Can you work these out from the model? Positions are in its coordinate system, mm. Face numbers are marked on the shaded views. Coordinates: 2 decimals unless noted, no trailing zeros. Write each loop counter-clockwise with the first axis right and the second up, starting at its lowest first coordinate (ties: lowest second). Pieces come first, ordered by that corner, then holes. Notation, with made-up numbers: (30, 29.5) -> (70, 29.5) arc R17 cw to (70, 56.5) -> close; hole circle Ø5 at (40, 20). An arc over 180 degrees is marked (long way). Use one line per item in the form item = value.
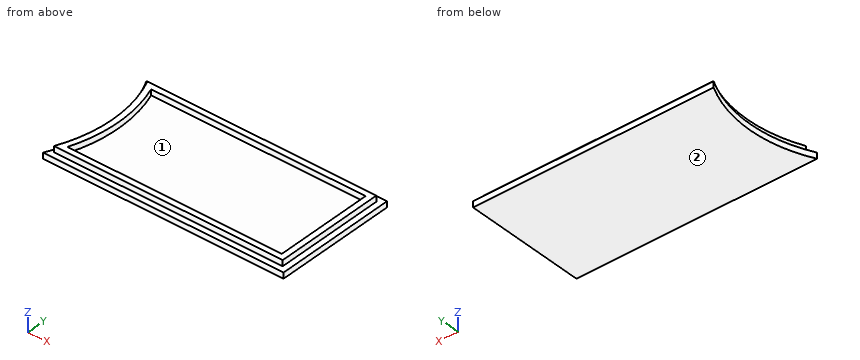
Autodesk Inventor part; units mm, degrees
ref_plane "YZ Plane" through (0, 0, 0) normal (1, 0, 0) x (0, 1, 0)
ref_plane "XZ Plane" through (0, 0, 0) normal (0, 1, 0) x (-1, 0, 0)
ref_plane "XY Plane" through (0, 0, 0) normal (0, 0, 1) x (1, 0, 0)
sketch "Sketch1" plane through (0, 0, 0) normal (0, 0, 1) x (1, 0, 0)
  circle A0 centre (0, 0) radius 45.75
  circle A1 centre (0, 0) radius 46.75
  line L0 (45.75, -0.0157) -> (46.75, -0.0157) construction
  line L1 (42.7149, 19) -> (121.75, 19)
  line L2 (121.75, 19) -> (121.75, -19)
  line L3 (121.75, -19) -> (42.7149, -19)
  line L4 (41.768, 21) -> (123.75, 21)
  line L5 (123.75, 21) -> (123.75, -21)
  line L6 (123.75, -21) -> (41.768, -21)
  line L7 (82.759, 21) -> (82.759, 19) construction
  line L8 (121.75, 0) -> (123.75, 0) construction
  line L9 (98.0367, -19) -> (98.0367, -21) construction
  line L10 (0, 0) -> (121.75, 0) construction
  line L11 (41.768, 21) -> (40.6456, 21)
  line L12 (41.768, -21) -> (40.6456, -21)
  line L13 (45.6899, 17) -> (119.75, 17)
  line L14 (119.75, 17) -> (119.75, -17)
  arc A2 (44.895, -19) -> (44.895, 19) centre (0, 0) ccw
  line L15 (119.75, -17) -> (45.6899, -17)
  dimension "d0" = 91.5
  dimension "d2" = 1
  dimension "d3" = 75
  dimension "d4" = 38
  dimension "d5" = 2
  dimension "d62" = 2
  dimension "d63" = 2
extrude "Extrusion13" add sketch "Sketch1" against normal blind 2 contours A0 L11 A1 L12 | L4 L5 L6 A1 L3 L2 L1 | L1 A2 L3 A1 | L1 L2 L3 A2 L15 L14 L13 | L13 L14 L15 A2 picked at (42.2726, -18.1004)
extrude "Extrusion14" add sketch "Sketch1" along normal blind 2 contours L1 A2 L3 A1 | L1 L2 L3 A2 L15 L14 L13
properties part number "Pump lid MM0312"
Q1. Will these pins go through, and if not, where does the flat tip stop? pin 1 (1 mm diameter, centred on x = 64.5, z = 1, fed in from -Y); pin 2 (12 mm diameter, centred on x = 105, y = 8, fed in from +Z); pin 3 (1.6 mm diameter, centred on y = -1, z = 1.5, fed in from -X).
Return value:
pin_1 = -19
pin_2 = 0
pin_3 = 46.72
Q2. Suppose I cut it at D-D (x = 48). Write out the boundary of the cut face in (y, z).
Return value:
outline = (-21, -2) -> (21, -2) -> (21, 0) -> (19, 0) -> (19, 2) -> (17, 2) -> (17, 0) -> (8.52, 0) -> (8.52, 2) -> (-8.52, 2) -> (-8.52, 0) -> (-17, 0) -> (-17, 2) -> (-19, 2) -> (-19, 0) -> (-21, 0) -> close
Q3. Suppose I cut it at A-A (x = 110). Write out the boundary of the cut face in (y, z).
Return value:
outline = (-21, -2) -> (21, -2) -> (21, 0) -> (19, 0) -> (19, 2) -> (17, 2) -> (17, 0) -> (-17, 0) -> (-17, 2) -> (-19, 2) -> (-19, 0) -> (-21, 0) -> close
Q4. Thinking about a two-plate mould opening in Y: for the marked faces 1 and 2, which applies, released by +Y, released by -Y, zero draft, split by the parting line, or undercut?
Return value:
face_1 = undercut
face_2 = zero draft
Q5. Suppose I cut it at C-C (y = 14.5). Write out the boundary of the cut face in (x, z), then the cut area to 3 significant figures.
Return value:
outline = (43.39, -2) -> (123.75, -2) -> (123.75, 0) -> (121.75, 0) -> (121.75, 2) -> (119.75, 2) -> (119.75, 0) -> (46.54, 0) -> (46.54, 2) -> (44.44, 2) -> (44.44, 0) -> (43.39, 0) -> close
area = 169 mm2
Q6. Suppose I cut it at B-B (z = 1.35). Write out the boundary of the cut face in (x, y), then the cut area to 3 significant figures.
Return value:
outline = (42.71, -19) -> (121.75, -19) -> (121.75, 19) -> (42.71, 19) arc R46.75 cw to start; hole (45.69, -17) -> (119.75, -17) -> (119.75, 17) -> (45.69, 17) arc R48.75 cw to start
area = 452 mm2
Q7. If I drill on line 1 (Y direction, x = 80.5, z = 1.05); line 2 (Z direction, x = 112, y = 5.5); line 3 (X direction, y = -16, z = 1.55), over which ranges is the centre line in solid material (lowest first)? Write a range as from..to.
Return value:
line_1 = -19..-17, 17..19
line_2 = -2..0
line_3 = 43.93..46.05, 119.75..121.75
